from build123d import *

# Parameters (mm, degrees)
BOSS_EXTRUDE1_DEPTH = 1
BOSS_EXTRUDE2_DEPTH = 2


with BuildPart() as part:
    # Sketch1 → Boss-Extrude1 (new body)
    with BuildSketch(Plane(origin=(0, 0, 0), x_dir=(1, 0, 0), z_dir=(0, 1, 0))):
        with BuildLine():
            Line((-3.175, 2.28), (3.175, 2.28))
            ThreePointArc((3.175, 2.28), (4.589213562, 1.694213562), (5.175, 0.28))
            Line((5.175, 0.28), (5.175, -0.28))
            ThreePointArc((5.175, -0.28), (4.589213562, -1.694213562), (3.175, -2.28))
            Line((3.175, -2.28), (-3.175, -2.28))
            ThreePointArc((-3.175, -2.28), (-4.589213562, -1.694213562), (-5.175, -0.28))
            Line((-5.175, -0.28), (-5.175, 0.28))
            ThreePointArc((-5.175, 0.28), (-4.589213562, 1.694213562), (-3.175, 2.28))
        make_face()
        with BuildLine():
            Line((-3.175, -1.28), (3.175, -1.28))
            ThreePointArc((3.175, -1.28), (3.882106781, -0.987106781), (4.175, -0.28))
            Line((4.175, -0.28), (4.175, 0.28))
            ThreePointArc((4.175, 0.28), (3.882106781, 0.987106781), (3.175, 1.28))
            Line((3.175, 1.28), (-3.175, 1.28))
            ThreePointArc((-3.175, 1.28), (-3.882106781, 0.987106781), (-4.175, 0.28))
            Line((-4.175, 0.28), (-4.175, -0.28))
            ThreePointArc((-4.175, -0.28), (-3.882106781, -0.987106781), (-3.175, -1.28))
        make_face(mode=Mode.SUBTRACT)
    extrude(amount=BOSS_EXTRUDE1_DEPTH)

    # Sketch1_2 → Boss-Extrude2 (add)
    with BuildSketch(Plane(origin=(0, 0, 0), x_dir=(1, 0, 0), z_dir=(0, 1, 0))):
        with BuildLine():
            ThreePointArc((3.175, 1.28), (3.882106781, 0.987106781), (4.175, 0.28))
            Line((4.175, 0.28), (4.175, -0.28))
            ThreePointArc((4.175, -0.28), (3.882106781, -0.987106781), (3.175, -1.28))
            Line((3.175, -1.28), (-3.175, -1.28))
            ThreePointArc((-3.175, -1.28), (-3.882106781, -0.987106781), (-4.175, -0.28))
            Line((-4.175, -0.28), (-4.175, 0.28))
            ThreePointArc((-4.175, 0.28), (-3.882106781, 0.987106781), (-3.175, 1.28))
            Line((-3.175, 1.28), (3.175, 1.28))
        make_face()
    extrude(amount=BOSS_EXTRUDE2_DEPTH)


solid = part.part
Design review of the part built by this model. Coordinates are the model's own, in mm. A direction names the side the tool comes from. Round coordinates to 2 decimals unless told otherwise and drop trailing zeros. Write each loop counter-clockwise with the first axis right and the second up, starting at its lowest first coordinate (ties: lowest second). Pieces come first, ordered by that corner, then holes. Notation, with made-up numbers: (-2.5, 58.25) -> (44.5, 58.25) arc R5 cw to (44.5, 66.25) -> close; hole circle Ø1 at (-17.5, 39.5). An arc over 180 degrees is marked (long way). One line per question, with ' | ' between items.
(1) Take a section at B-B, the plane z = -0.1. State the section outline as (x, y) points (3 decimals), and give its area (3 significant figures).
Result sheet:
outline: (-5.175, 0) -> (5.175, 0) -> (5.175, 1) -> (4.175, 1) -> (4.175, 2) -> (-4.175, 2) -> (-4.175, 1) -> (-5.175, 1) -> close | area: 18.7 mm2
(2) Take a section at A-A, the plane x = 1.5. State the section outline as (y, z) points, and give its area (3 significant figures).
Result sheet:
outline: (0, -2.28) -> (1, -2.28) -> (1, -1.28) -> (2, -1.28) -> (2, 1.28) -> (1, 1.28) -> (1, 2.28) -> (0, 2.28) -> close | area: 7.12 mm2
(3) Wall thickness on line 1 (Z direction, x = -3.25, y = 1.75); line 2 (X direction, y = 1.1, z = 0) (3 decimals); line 3 (Y direction, x = -0.5, z = 1.8): over which ranges is each line inside the solid? List them lowest first. Write a range as [from, to].
Result sheet:
line 1: [-1.28, 1.28] | line 2: [-4.175, 4.175] | line 3: [0, 1]
(4) Take a section at C-C, the plane z = 1.7. State the section outline as (x, y) points.
Result sheet:
outline: (-4.58, 0) -> (4.58, 0) -> (4.58, 1) -> (-4.58, 1) -> close
(5) Insertion check: P1, Ø0.6, axis at y = 1.5, z = 0, coming from the +X side (3 decimals); P2, Ø0.6, axis at y = 1.5, z = 0, coming from the -X side (3 decimals); P3, Ø0.5, axis at x = -1, y = 1.5, coming from the +Z side. Each pin has a flat end and moves straight along its axis. Give the tip position at first contact, or say it passes through.
Result sheet:
P1: x = 4.175 | P2: x = -4.175 | P3: z = 1.28
(6) Machinability: for faces 1 (the cylindrical face through (3.89, 1.49, 0.98)), 2 (the flat face through (0, 1.5, -1.28)), 3 (the cylindrical face through (-3.89, 1.49, -0.98)), 4 (the cylindrical face through (-3.874, 1.493, 0.995)), 5 (the cylindrical face through (3.874, 1.493, -0.995)), which of the approach directions +Z, -Z, +X, -X, +Y, -Y give a long, thin tool a straight path to every point of the face, cutting with its end or side? Answer none if there is none.
Result sheet:
face 1: +Z, +X, +Y | face 2: -Z, +X, -X, +Y | face 3: -Z, -X, +Y | face 4: +Z, -X, +Y | face 5: -Z, +X, +Y
